Design review of the part built by this model. Coordinates are the model's own, in mm. A direction names the side the tool comes from. Coordinates: 2 decimals unless noted, no trailing zeros. Loops run counter-clockwise (first coordinate to the right, second up) from the corner with the lowest first, then second, coordinate; pieces in that order, holes last. Notation, with made-up numbers: M 63.5,36 L 121.5,36 A23 cw 121.5,55 Z; hole C 72.5,-21.5 d5. An arc over 180 degrees is marked long. Put each result on its own line as item: value. Start each with the question number.
(1) Take a section at C-C, the plane x = -27. Give the boundary of the cut face in (y, z), then the cut area to 3 significant figures.
(2) Clearance check with flat-ended pins moving along their axes: pin 1 (2.5 mm diameter, centred on x = -35.32, y = -15.5, fed in from -Z); pin 2 (0.8 mm diameter, centred on y = 6, z = 1.5, fed in from -X); pin 3 (0.8 mm diameter, centred on x = -14, z = 1.5, fed in from -Y); pin 4 (1.5 mm diameter, centred on x = -16, z = 1.5, fed in from +Y). State where each tip first meets the part, or that it passes through.
(3) Take a section at D-D, the plane z = 0.75. Count the separate pieces of the cut face and the enclosed holes in it, then the cut area to 3 significant figures.
(4) Take a section at B-B, the plane y = 15.5. Give the boundary of the cut face in (x, z).
(5) For probe 1 along Y at (x, z) = (-14, 2.2); probe 2 along Y at (x, z) = (46.5, 1.2); probe 3 along X at (y, z) = (9, 1.55), list the stretches that pass through material, from the lowest coordinate up. Write a range as [from, to].
(6) Take a section at A-A, the plane x = 83. Give the boundary of the cut face in (y, z).
(7) For faces 5 (the cylindrical face through (29.81, -20.603, 1.232)), 6 (the cylindrical face through (23.08, 6.17, 1.23)), 7 (the flat face through (36, 20, 1)), list the 3-axis set-ups (+Z, -Z, +X, -X, +Y, -Y) from which the entire face can be reached by the end or side of a thin tool; tool diameter is ignored.
(8) The part is to be moulded in two halves that separate along X. For faces 1 (the cylindrical face through (-19.263, 4.975, 1.232)), 2 (the flat face through (15, 20, 1)), 3 (the flat face through (56, 24, 1)), 4 (the cylindrical face through (113.848, -8.651, 1.232)), say which applies: +X half, -X half, draft (parallel to the pull), parting line (faces both ways), or undercut.
```python
from build123d import *

# Parameters (mm, degrees)
CROQUIS1_R              = 1.5
SALIENTE_EXTRUIR1_DEPTH = 2.5


with BuildPart() as part:
    # Croquis1 → Saliente-Extruir1 (new body)
    with BuildSketch(Plane.XY):
        with BuildLine():
            Line((-1.727869, -20), (-35.318076, -20))
            ThreePointArc((-35.318076, -20), (-39.801686502, -15.883714562), (-36.082710062, -11.065438607))
            add(Edge.make_bspline(
                [(-36.082710062, -11.065438607), (-34.968163592, -10.873261807), (-33.318075526, -9.571810644), (-33.318075526, -8.000000003)],
                knots=[0, 0, 0, 0, 1, 1, 1, 1], degree=3))
            Line((-33.318075526, -8.000000003), (-33.318076, 0))
            Line((-33.318076, 0), (-33.318075526, 7.999999997))
            add(Edge.make_bspline(
                [(-36.082710062, 11.065438607), (-34.968163592, 10.873261801), (-33.318075526, 9.571810638), (-33.318075526, 7.999999997)],
                knots=[0, 0, 0, 0, 1, 1, 1, 1], degree=3))
            ThreePointArc((-36.082710062, 11.065438607), (-39.801686502, 15.883714562), (-35.318076, 20))
            Line((-35.318076, 20), (-1.727869, 20))
            ThreePointArc((-1.727869, 20), (0.410220921, 20.619382972), (1.886162597, 22.285714256))
            ThreePointArc((1.886162597, 22.285714256), (2.993118801, 23.535462608), (4.596686131, 23.999999793))
            Line((4.596686131, 23.999999793), (17.855013131, 23.999999793))
            ThreePointArc((17.855013131, 23.999999793), (18.20856652, 23.93541414), (18.516450957, 23.749999795))
            ThreePointArc((18.516450957, 23.749999795), (19.177888957, 23.499999641), (19.839326957, 23.749999792))
            ThreePointArc((19.839326957, 23.749999792), (20.147211189, 23.935413861), (20.500764274, 23.999999414))
            Line((20.500764274, 23.999999414), (25.596686274, 23.999999414))
            ThreePointArc((25.596686274, 23.999999414), (27.200253319, 23.535462249), (28.307209321, 22.285714093))
            ThreePointArc((28.307209321, 22.285714093), (29.783150997, 20.61938281), (31.921240919, 19.999999837))
            Line((31.921240919, 19.999999837), (39.272130919, 19.999999837))
            ThreePointArc((39.272130919, 19.999999837), (41.41022084, 20.61938281), (42.886162516, 22.285714093))
            ThreePointArc((42.886162516, 22.285714093), (43.993118719, 23.535462445), (45.596686049, 23.999999631))
            Line((45.596686049, 23.999999631), (66.596686049, 23.999999631))
            ThreePointArc((66.596686049, 23.999999631), (68.20025338, 23.535462445), (69.307209583, 22.285714093))
            ThreePointArc((69.307209583, 22.285714093), (70.783151259, 20.61938281), (72.92124118, 19.999999837))
            Line((72.92124118, 19.999999837), (107.61258818, 19.999999837))
            ThreePointArc((107.61258818, 19.999999837), (110.006914096, 19.249811631), (111.545093682, 17.267494173))
            ThreePointArc((111.545093682, 17.267494173), (113.827321184, 8.772458491), (114.473968889, -7.06e-07))
            ThreePointArc((114.473968889, -7.06e-07), (113.827321261, -8.772459139), (111.545094118, -17.267494122))
            ThreePointArc((111.545094118, -17.267494122), (110.006914516, -19.249811879), (107.612588369, -20.000000175))
            Line((107.612588369, -20.000000175), (72.921241369, -20.000000175))
            ThreePointArc((72.921241369, -20.000000175), (70.783151447, -20.619383147), (69.307209771, -22.285714431))
            ThreePointArc((69.307209771, -22.285714431), (68.200253515, -23.535462843), (66.596686107, -24.000000051))
            Line((66.596686107, -24.000000051), (45.596686107, -24.000000051))
            ThreePointArc((45.596686107, -24.000000051), (43.993118827, -23.535462721), (42.886162705, -22.285714307))
            ThreePointArc((42.886162705, -22.285714307), (41.410221028, -20.619383023), (39.272131107, -20.000000051))
            Line((39.272131107, -20.000000051), (31.921241107, -20.000000051))
            ThreePointArc((31.921241107, -20.000000051), (29.783151186, -20.619383023), (28.30720951, -22.285714307))
            ThreePointArc((28.30720951, -22.285714307), (27.200253316, -23.535462648), (25.596686, -23.999999829))
            Line((25.596686, -23.999999829), (20.500764, -23.999999829))
            ThreePointArc((20.500764, -23.999999829), (20.14721061, -23.935414176), (19.839326174, -23.74999983))
            ThreePointArc((19.839326174, -23.74999983), (19.177888468, -23.50000009), (18.516450826, -23.750000001))
            ThreePointArc((18.516450826, -23.750000001), (18.20856639, -23.935414347), (17.855013, -24))
            Line((17.855013, -24), (4.596686, -24))
            ThreePointArc((4.596686, -24), (2.993118559, -23.535462771), (1.886162302, -22.285714308))
            ThreePointArc((1.886162302, -22.285714308), (0.410220761, -20.619383073), (-1.727869, -20))
        make_face()
        with Locations((107.612588, -15.5)):
            Circle(CROQUIS1_R, mode=Mode.SUBTRACT)
        with Locations((-35.318076, -15.5)):
            Circle(CROQUIS1_R, mode=Mode.SUBTRACT)
        with Locations((-35.318076, 15.5)):
            Circle(CROQUIS1_R, mode=Mode.SUBTRACT)
        with Locations((107.612588, 15.5)):
            Circle(CROQUIS1_R, mode=Mode.SUBTRACT)
        with BuildLine():
            Line((66.596686049, 19.999999775), (45.596686049, 19.999999775))
            ThreePointArc((45.596686049, 19.999999775), (44.596686049, 20.999999775), (45.596686049, 21.999999775))
            Line((45.596686049, 21.999999775), (66.596686049, 21.999999775))
            ThreePointArc((66.596686049, 21.999999775), (67.596686049, 20.999999775), (66.596686049, 19.999999775))
        make_face(mode=Mode.SUBTRACT)
        with BuildLine():
            Line((4.596686131, 21.999999938), (25.596686131, 21.999999938))
            ThreePointArc((25.596686131, 21.999999938), (26.596686131, 20.999999938), (25.596686131, 19.999999938))
            Line((25.596686131, 19.999999938), (4.596686131, 19.999999938))
            ThreePointArc((4.596686131, 19.999999938), (3.596686131, 20.999999938), (4.596686131, 21.999999938))
        make_face(mode=Mode.SUBTRACT)
        with BuildLine():
            Line((60.629579, -4.165983), (98.473924, -4.165983))
            ThreePointArc((98.473924, -4.165983), (100.546598144, -4.997118122), (101.470828647, -7.029988427))
            ThreePointArc((101.470828647, -7.029988427), (99.46254802, -11.787003007), (94.502482097, -13.222316504))
            ThreePointArc((94.502482097, -13.222316504), (78.165345659, -10.947800594), (61.735508446, -9.48632916))
            ThreePointArc((61.735508446, -9.48632916), (60.624439263, -9.309527068), (59.565908087, -8.928416245))
            ThreePointArc((59.565908087, -8.928416245), (58.189693438, -6.121044064), (60.629579, -4.165983))
        make_face(mode=Mode.SUBTRACT)
        with BuildLine():
            Line((25.596686, -20), (4.596686, -20))
            ThreePointArc((4.596686, -20), (3.596686, -21), (4.596686, -22))
            Line((4.596686, -22), (25.596686, -22))
            ThreePointArc((25.596686, -22), (26.596686, -21), (25.596686, -20))
        make_face(mode=Mode.SUBTRACT)
        with BuildLine():
            Line((66.596686107, -20.000000051), (45.596686107, -20.000000051))
            ThreePointArc((45.596686107, -20.000000051), (44.596686427, -21.000000051), (45.596686107, -22.000000051))
            Line((45.596686107, -22.000000051), (66.596686107, -22.000000051))
            ThreePointArc((66.596686107, -22.000000051), (67.596686107, -21.000000051), (66.596686107, -20.000000051))
        make_face(mode=Mode.SUBTRACT)
        with BuildLine():
            Line((20.630693, -4.165983), (-17.213652, -4.165983))
            ThreePointArc((-17.213652, -4.165983), (-19.286331958, -4.997112835), (-20.210567815, -7.029984473))
            ThreePointArc((-20.210567815, -7.029984473), (-18.202285238, -11.787004738), (-13.242211847, -13.222314))
            ThreePointArc((-13.242211847, -13.222314), (3.094925006, -10.947797585), (19.524762662, -9.486325691))
            ThreePointArc((19.524762662, -9.486325691), (20.635832812, -9.309527332), (21.694365632, -8.928419991))
            ThreePointArc((21.694365632, -8.928419991), (23.070588154, -6.121043634), (20.630693, -4.165983))
        make_face(mode=Mode.SUBTRACT)
        with BuildLine():
            Line((60.629579, 4.165983), (98.473924, 4.165983))
            ThreePointArc((98.473924, 4.165983), (100.546603429, 4.997112019), (101.470840047, 7.029982437))
            ThreePointArc((101.470840047, 7.029982437), (99.462556799, 11.787003808), (94.502482022, 13.222312881))
            ThreePointArc((94.502482022, 13.222312881), (78.165344631, 10.947798744), (61.735506549, 9.486329166))
            ThreePointArc((61.735506549, 9.486329166), (60.624437652, 9.309528853), (59.565906368, 8.928419991))
            ThreePointArc((59.565906368, 8.928419991), (58.189683846, 6.121043634), (60.629579, 4.165983))
        make_face(mode=Mode.SUBTRACT)
        with BuildLine():
            Line((20.630693, 4.165983), (-17.213652, 4.165983))
            ThreePointArc((-17.213652, 4.165983), (-19.286325559, 4.99711656), (-20.210557539, 7.029984958))
            ThreePointArc((-20.210557539, 7.029984958), (-18.202276912, 11.786999538), (-13.242210989, 13.222313035))
            ThreePointArc((-13.242210989, 13.222313035), (3.094925937, 10.947798842), (19.524763554, 9.48632916))
            ThreePointArc((19.524763554, 9.48632916), (20.635832737, 9.309527068), (21.694363913, 8.928416245))
            ThreePointArc((21.694363913, 8.928416245), (23.070578562, 6.121044064), (20.630693, 4.165983))
        make_face(mode=Mode.SUBTRACT)
    extrude(amount=SALIENTE_EXTRUIR1_DEPTH)


solid = part.part
```
Computed values:
1. outline: M -20,0 L 20,0 L 20,2.5 L -20,2.5 Z
1. area: 100 mm^2
2. pin 1: passes through
2. pin 2: stops at x = -33.32
2. pin 3: stops at y = -20
2. pin 4: stops at y = 20
3. separate pieces: 1
3. enclosed holes: 12
3. area: 5,000 mm^2
4. outline: M -39.82,0 L -36.82,0 L -36.82,2.5 L -39.82,2.5 Z; M -33.82,0 L 106.11,0 L 106.11,2.5 L -33.82,2.5 Z; M 109.11,0 L 112.16,0 L 112.16,2.5 L 109.11,2.5 Z
5. probe 1: y = [-20, -13.3], [-4.17, 4.17], [13.3, 20]
5. probe 2: y = [-24, -22], [-20, 20], [22, 24]
5. probe 3: x = [-33.54, -19.97], [21.54, 59.72], [101.23, 113.79]
6. outline: M -20,0 L -11.53,0 L -11.53,2.5 L -20,2.5 Z; M -4.17,0 L 4.17,0 L 4.17,2.5 L -4.17,2.5 Z; M 11.53,0 L 20,0 L 20,2.5 L 11.53,2.5 Z
7. face 5: +Z, -Z, -Y
7. face 6: +Z, -Z
7. face 7: +Z, -Z, +Y
8. face 1: undercut
8. face 2: undercut
8. face 3: draft
8. face 4: +X half
